Geometry check sheet. Reference: the model listing, model coordinates, mm. A direction names the side the tool comes from. Give positions to 0.01 mm unless a question says otherwise; leave off trailing zeros. Write each loop counter-clockwise with the first axis right and the second up, starting at its lowest first coordinate (ties: lowest second). Pieces come first, ordered by that corner, then holes. Notation, with made-up numbers: (-36, -33) - (14, -33) arc R19 cw to (14, -22) - close; hole circle Ø8 at (-33, -3). An arc over 180 degrees is marked (long way). Use a Markdown table: item, result.
```python
from build123d import *

# Parameters (mm, degrees)
F1_DEPTH = 65
F2_W     = 100
F2_H     = 60
F3_DEPTH = 265
F4_R     = 15
F5_DEPTH = 265


with BuildPart() as f1:
    # F0 (on Right) → F1 (new body, symmetric)
    with BuildSketch(Plane.YZ):
        Polygon((0, 250), (0, 0), (1200, 0), (1200, 1280), (1120, 1280), (1120, 150), (820, 150), (820, 250), (288.740796, 392.350475), (181.595789, 1000), (-18.404211, 1000), (-18.404211, 880), (134.056628, 808.906343), (218.578984, 329.556244), align=None)
    extrude(amount=F1_DEPTH, both=True)

    # F2 (on Right) → F3 (join, symmetric)
    with BuildSketch(Plane.YZ):
        with Locations((50, 30)):
            Rectangle(F2_W, F2_H)
        with Locations((1150, 30)):
            Rectangle(F2_W, F2_H)
    extrude(amount=F3_DEPTH, both=True)

    # F4 (on Right) → F5 (join, symmetric)
    with BuildSketch(Plane.YZ):
        with Locations((1170, 1030)):
            Circle(F4_R)
    extrude(amount=F5_DEPTH, both=True)


solid = f1.part
```
1) Section check A-A on x = 34. Record the boundary of the cut face in (y, z).
Working result:
| item | result |
|---|---|
| outline | (-18.4, 880) - (134.06, 808.91) - (218.58, 329.56) - (0, 250) - (0, 0) - (1200, 0) - (1200, 1280) - (1120, 1280) - (1120, 150) - (820, 150) - (820, 250) - (288.74, 392.35) - (181.6, 1000) - (-18.4, 1000) - close |
2) Section check B-B on x = 161. Record the boundary of the cut face in (y, z), then the cut area to 3 significant figures.
Working result:
| item | result |
|---|---|
| outline | (0, 0) - (100, 0) - (100, 60) - (0, 60) - close; (1100, 0) - (1200, 0) - (1200, 60) - (1100, 60) - close; circle Ø30 at (1170, 1030) |
| area | 12,700 mm² |
3) Set-up check for faces 1 (the cylindrical face through (-163.6, 1184.307, 1034.506)), 2 (the flat face through (-164, 1100, 30)), 3 (the cylindrical face through (166.4, 1184.307, 1034.506)), 4 (the flat face through (4, 0, 99)), 5 (the flat face through (164, 100, 30)): record each of +Z, -Z, +X, -X, +Y, -Y from which the full face is reachable in a straight line by a thin tool's end or side.
Working result:
| item | result |
|---|---|
| face 1 | -X |
| face 2 | +Z, -Z, -X |
| face 3 | +X |
| face 4 | -Z, +X, -X, -Y |
| face 5 | +Z, -Z, +X |
4) Depth check by flat-ended pin: P1, Ø1.5, axis at x = -33, z = 480.5, coming from the -Y side. Enter the tip coordinate at first touch or a pass-through.
Working result:
| item | result |
|---|---|
| P1 | stops at y = 191.83 |
5) Section check D-D on y = 1170. Record the boundary of the cut face in (x, z), then the cut area to 3 significant figures.
Working result:
| item | result |
|---|---|
| outline | (-265, 0) - (265, 0) - (265, 60) - (65, 60) - (65, 1015) - (265, 1015) - (265, 1045) - (65, 1045) - (65, 1280) - (-65, 1280) - (-65, 1045) - (-265, 1045) - (-265, 1015) - (-65, 1015) - (-65, 60) - (-265, 60) - close |
| area | 202,000 mm² |
6) Material ranges on L1, parallel to X at y = 152.5, z = 214.5; L2, parallel to Y at x = 54, z = 1009; L3, parallel to Y at x = 4.5, z = 896, recorded low to high. Write a range as from..to.
Working result:
| item | result |
|---|---|
| L1 | x = -65..65 |
| L2 | y = 1120..1200 |
| L3 | y = -18.4..199.93, 1120..1200 |
7) Section check C-C on z = 744.5. Record the boundary of the cut face in (x, y), then the cut area to 3 significant figures.
Working result:
| item | result |
|---|---|
| outline | (-65, 145.41) - (65, 145.41) - (65, 226.65) - (-65, 226.65) - close; (-65, 1120) - (65, 1120) - (65, 1200) - (-65, 1200) - close |
| area | 21,000 mm² |
8) Mould release check, pull along Z, two halves, no side actions. Record for faces 6 (the flat face through (0.91, 110.82, 290.335)), 7 (the flat face through (-265, 1170, 1030)), 8 (the flat face through (164, 49, 60)): pulls with the +Z half, pulls with the -Z half, needs draft (parallel to the pull), parting line crosses it, or undercut.
Working result:
| item | result |
|---|---|
| face 6 | undercut |
| face 7 | needs draft |
| face 8 | pulls with the +Z half |
